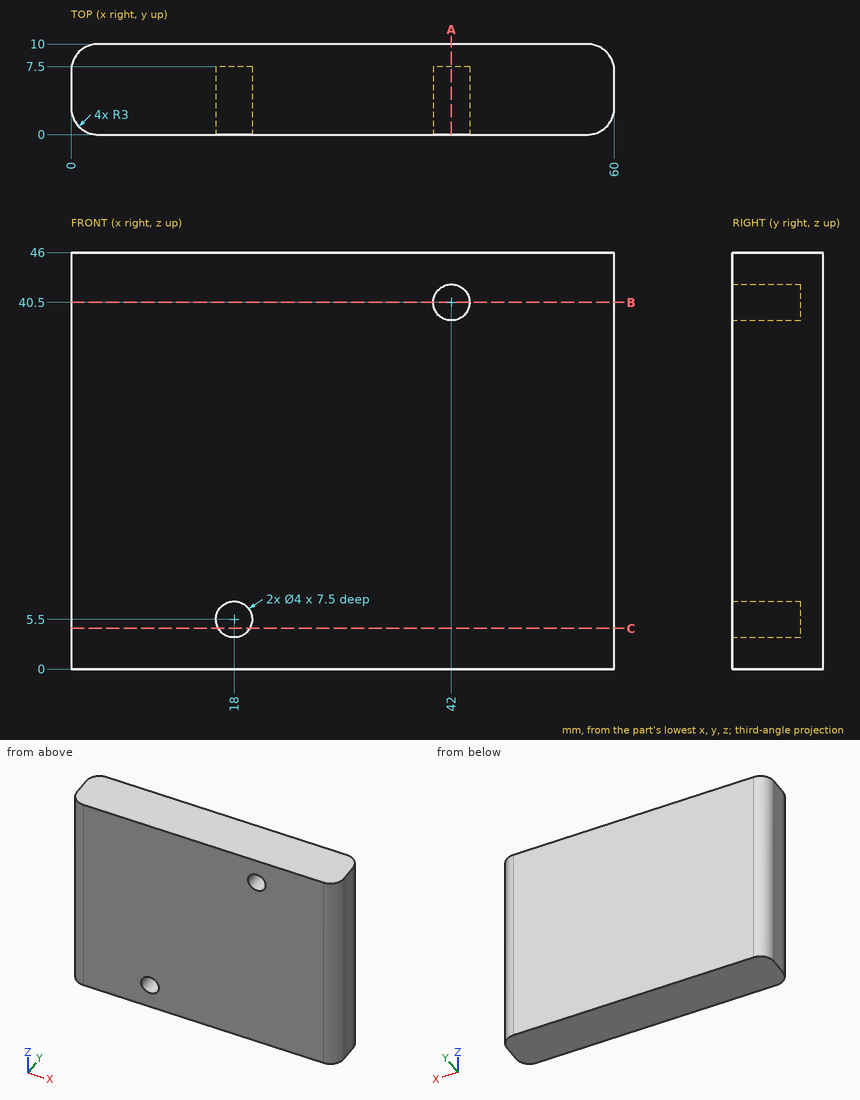
Job drawing, mm, ordinate dimensions from the low corner. One solid piece. Coordinates: 2 decimals unless noted, no trailing zeros. Order: outer loops, then holes, each group sorted by start corner. A loop starts at its lowest first (then second) coordinate and runs counter-clockwise, first axis right, second up. Notation, with made-up numbers: M -14,39 L 31,39 A17 cw 31,55 Z; hole C -37.5,40.25 d7. An arc over 180 degrees is marked long. Answer as CSV lines item,"result".
(1) Band-saw the part on B-B, the plane z = 40.5. List the corners of the cut face in (x, y), then the cut area to 3 significant figures.
Geometry says:
outline,"M 0,3 A3 ccw 3,0 L 40,0 L 40,7.5 L 44,7.5 L 44,0 L 57,0 A3 ccw 60,3 L 60,7 A3 ccw 57,10 L 3,10 A3 ccw 0,7 Z"
area,"562 mm2"
(2) Band-saw the part on C-C, the plane z = 4.5. List the corners of the cut face in (x, y).
Geometry says:
outline,"M 0,3 A3 ccw 3,0 L 16.27,0 L 16.27,7.5 L 19.73,7.5 L 19.73,0 L 57,0 A3 ccw 60,3 L 60,7 A3 ccw 57,10 L 3,10 A3 ccw 0,7 Z"
(3) Band-saw the part on A-A, the plane x = 42. List the corners of the cut face in (y, z), then the cut area to 3 significant figures.
Geometry says:
outline,"M 0,0 L 10,0 L 10,46 L 0,46 L 0,42.5 L 7.5,42.5 L 7.5,38.5 L 0,38.5 Z"
area,"430 mm2"
(4) Flat gauge pin, fed straight in: pin 1 (2 mm diameter, centred on x = 42, z = 40, fed in from -Y). Where does the tip first touch, or does it go through?
Geometry says:
pin 1,"stops at y = 7.5"
(5) Wall check: line 1 along X through (y, z) = (5.5, 5.5); line 2 along Z through (x, y) = (19, 4.5); line 3 along X through (y, z) = (2, 5.5). Give the ranges that are in metal, low to high.
Geometry says:
line 1,"x = 0 to 16, 20 to 60"
line 2,"z = 0 to 3.77, 7.23 to 46"
line 3,"x = 0.17 to 16, 20 to 59.83"
